from build123d import *

# Parameters (mm, degrees)
ESQUISSE1_W             = 36
ESQUISSE1_H             = 6
BOSS_EXTRU_1_DEPTH      = 6
ESQUISSE2_R             = 1.5
ENL_V_MAT_EXTRU_1_DEPTH = 60
ESQUISSE3_R             = 1.5
ENL_V_MAT_EXTRU_2_DEPTH = 6


with BuildPart() as part:
    # Esquisse1 → Boss.-Extru.1 (new body)
    with BuildSketch(Plane(origin=(0, 0, 0), x_dir=(1, 0, 0), z_dir=(0, 1, 0))):
        Rectangle(ESQUISSE1_W, ESQUISSE1_H)
    extrude(amount=BOSS_EXTRU_1_DEPTH)

    # Esquisse2 → Enlèv. mat.-Extru.1 (cut)
    with BuildSketch(Plane(origin=(0, 6, 0), x_dir=(1, 0, 0), z_dir=(0, 1, 0))):
        with Locations((-15, 0)):
            Circle(ESQUISSE2_R)
    enl_v_mat_extru_1 = extrude(amount=-ENL_V_MAT_EXTRU_1_DEPTH, mode=Mode.SUBTRACT)

    # Symétrie1: Enlèv. mat.-Extru.1 across plane
    add(enl_v_mat_extru_1.mirror(Plane(origin=(0, 0, 0), x_dir=(0, 0, 1), z_dir=(1, 0, 0))), mode=Mode.SUBTRACT)

    # Esquisse3 → Enlèv. mat.-Extru.2 (cut)
    with BuildSketch(Plane.XY.offset(3)):
        with Locations((-10.5, 3)):
            Circle(ESQUISSE3_R)
    enl_v_mat_extru_2 = extrude(amount=-ENL_V_MAT_EXTRU_2_DEPTH, mode=Mode.SUBTRACT)

    # Symétrie2: Enlèv. mat.-Extru.2 across plane
    add(enl_v_mat_extru_2.mirror(Plane(origin=(0, 0, 0), x_dir=(0, 0, 1), z_dir=(1, 0, 0))), mode=Mode.SUBTRACT)


solid = part.part
The model under review builds one solid part; all positions refer to its coordinate system, in mm. Coordinates: 2 decimals unless noted, no trailing zeros. Loops run counter-clockwise (first coordinate to the right, second up) from the corner with the lowest first, then second, coordinate; pieces in that order, holes last.
(1) Draft analysis for pull direction Z (two halves, no side actions). For faces 1 (the flat face through (0, 3, 3)), 2 (the cylindrical face through (-16.5, 3.04, -0.07)), 3 (the flat face through (0, 0, 0)), state which applies: +Z half, -Z half, draft (parallel to the pull), parting line (faces both ways), or undercut.
Determined:
face 1: +Z half
face 2: undercut
face 3: draft
(2) Insertion check: P1, Ø2.5, axis at x = -10.5, y = 3, coming from the -Z side. The pin has a flat end and moves straight along its axis. Give the tip position at first contact, or say it passes through.
Determined:
P1: passes through
(3) Consider section A-A, the plane x = 15. Give the boundary of the cut face in (y, z).
Determined:
outline: (0, -3) - (6, -3) - (6, -1.5) - (0, -1.5) - close; (0, 1.5) - (6, 1.5) - (6, 3) - (0, 3) - close
(4) Consider section B-B, the plane z = 0. Give the boundary of the cut face in (x, y).
Determined:
outline: (-18, 0) - (-16.5, 0) - (-16.5, 6) - (-18, 6) - close; (-13.5, 0) - (13.5, 0) - (13.5, 6) - (-13.5, 6) - close; (16.5, 0) - (18, 0) - (18, 6) - (16.5, 6) - close; hole circle Ø3 at (-10.5, 3); hole circle Ø3 at (10.5, 3)
(5) Consider section D-D, the plane y = 0.5. Give the boundary of the cut face in (x, z), plus the area to 3 significant figures.
Determined:
outline: (-18, -3) - (18, -3) - (18, 3) - (-18, 3) - close; hole circle Ø3 at (-15, 0); hole circle Ø3 at (15, 0)
area: 202 mm2
(6) Consider section C-C, the plane y = 1.95. Give the boundary of the cut face in (x, z).
Determined:
outline: (-18, -3) - (-11.57, -3) - (-11.57, 3) - (-18, 3) - close; (-9.43, -3) - (9.43, -3) - (9.43, 3) - (-9.43, 3) - close; (11.57, -3) - (18, -3) - (18, 3) - (11.57, 3) - close; hole circle Ø3 at (-15, 0); hole circle Ø3 at (15, 0)
(7) Wall thickness on L1, parallel to X at y = 4.6, z = 0; L2, parallel to Y at x = -10.5, z = -1.35; L3, parallel to X at y = 3.3, z = 0: over which ranges is each line inside the solid? List them lowest first.
Determined:
L1: x = -18 to -16.5, -13.5 to 13.5, 16.5 to 18
L2: y = 0 to 1.5, 4.5 to 6
L3: x = -18 to -16.5, -13.5 to -11.97, -9.03 to 9.03, 11.97 to 13.5, 16.5 to 18
